Autodesk Inventor part; units mm, degrees
ref_plane "Work Plane1" through (-39.4462, 0, -3.175) normal (0, 0, -1) x (0, 1, 0)
ref_plane "YZ Plane" through (0, 0, 0) normal (1, 0, 0) x (0, 1, 0)
ref_plane "XZ Plane" through (0, 0, 0) normal (0, 1, 0) x (-1, 0, 0)
sketch "Sketch1" plane through (0, 0, 0) normal (0, 0, 1) x (1, 0, 0)
  line L0 (-43.688, 0) -> (-43.688, 415.3)
  line L1 (0, 0) -> (0, 415.3)
  circle A0 centre (-7.6009, 150.0066) radius 1.1
  circle A1 centre (-13.6588, 173.1577) radius 6.4135
  circle A2 centre (-13.6588, 134.9467) radius 6.4135
  circle A3 centre (-7.6009, 188.2176) radius 1.1
  circle A4 centre (-7.6009, 92.9676) radius 1.1
  circle A5 centre (-13.6588, 245.4367) radius 6.4135
  circle A6 centre (-13.6588, 77.9077) radius 6.4135
  circle A7 centre (-7.6009, 260.4966) radius 1.1
  circle A8 centre (-7.6009, 54.7566) radius 1.1
  circle A9 centre (-13.6588, 283.6477) radius 6.4135
  circle A10 centre (-13.6588, 39.6967) radius 6.4135
  circle A11 centre (-7.6009, 298.7076) radius 1.1
  line L2 (-7.3698, 0) -> (-7.3698, 12.7)
  line L3 (-7.3698, 0) -> (-36.3182, 0)
  line L4 (-36.3182, 0) -> (-36.3182, 12.7)
  line L5 (-36.3182, 12.7) -> (-39.4462, 12.7)
  line L6 (-39.4462, 12.7) -> (-39.4462, 402.6)
  line L7 (-39.4462, 402.6) -> (-36.3182, 402.6)
  line L8 (-36.3182, 402.6) -> (-36.3182, 415.3)
  line L9 (-36.3182, 415.3) -> (-7.3698, 415.3)
  line L10 (-7.3698, 402.6) -> (-7.3698, 415.3)
  line L11 (-7.3698, 402.6) -> (-4.2418, 402.6)
  line L12 (-4.2418, 402.6) -> (-4.2418, 12.7)
  line L13 (-4.2418, 12.7) -> (-7.3698, 12.7)
  circle A12 centre (-13.6588, 340.6867) radius 6.4135
  circle A13 centre (-7.6009, 355.7466) radius 1.1
  circle A14 centre (-13.6588, 378.8977) radius 6.4135
  circle A15 centre (-34.9052, 110.3753) radius 3.2004
  circle A16 centre (-34.9052, 316.1153) radius 3.2004
  circle A17 centre (-7.6009, 393.9576) radius 1.1
  circle A18 centre (-11.9075, 15.1253) radius 3.302
  circle A19 centre (-23.6029, 54.7566) radius 1.1
  circle A20 centre (-23.6029, 92.9676) radius 1.1
  circle A21 centre (-23.6029, 188.2176) radius 1.1
  circle A22 centre (-23.6029, 260.4966) radius 1.1
  circle A23 centre (-34.9052, 322.1732) radius 1.1
  circle A24 centre (-23.6029, 355.7466) radius 1.1
  circle A25 centre (-23.6029, 393.9576) radius 1.1
  circle A26 centre (-23.6029, 298.7076) radius 1.1
  circle A27 centre (-23.6029, 150.0066) radius 1.1
  circle A28 centre (-34.9052, 116.4332) radius 1.1
  circle A29 centre (-11.9075, 316.1153) radius 3.302
  circle A30 centre (-13.6588, 328.1211) radius 3.302
  circle A31 centre (-13.6588, 366.3321) radius 3.302
  circle A32 centre (-13.6588, 271.0821) radius 3.302
  circle A33 centre (-13.6588, 232.8711) radius 3.302
  circle A34 centre (-29.6608, 160.5921) radius 3.302
  circle A35 centre (-29.6608, 122.3811) radius 3.302
  circle A36 centre (-11.9075, 110.3753) radius 3.302
  circle A37 centre (-13.6588, 65.3421) radius 3.302
  circle A38 centre (-13.6588, 27.1311) radius 3.302
  circle A39 centre (-29.6608, 27.1311) radius 3.302
  circle A40 centre (-29.6608, 65.3421) radius 3.302
  circle A41 centre (-13.6588, 122.3811) radius 3.302
  circle A42 centre (-13.6588, 160.5921) radius 3.302
  circle A43 centre (-11.9075, 220.8653) radius 3.302
  circle A44 centre (-29.6608, 232.8711) radius 3.302
  circle A45 centre (-29.6608, 271.0821) radius 3.302
  circle A46 centre (-29.6608, 366.3321) radius 3.302
  circle A47 centre (-29.6608, 328.1211) radius 3.302
  circle A48 centre (-29.6583, 340.6867) radius 6.4135
  circle A49 centre (-29.6583, 378.8977) radius 6.4135
  circle A50 centre (-29.6583, 245.4367) radius 6.4135
  circle A51 centre (-29.6583, 173.1577) radius 6.4135
  circle A52 centre (-29.6583, 134.9467) radius 6.4135
  circle A53 centre (-29.6583, 39.6967) radius 6.4135
  circle A54 centre (-29.6583, 77.9077) radius 6.4135
  circle A55 centre (-29.6583, 283.6477) radius 6.4135
  circle A56 centre (-22.9108, 110.3753) radius 4.5
  circle A57 centre (-22.9108, 220.8653) radius 4.5
  circle A58 centre (-22.9108, 316.1153) radius 4.5
  circle A59 centre (-13.6588, 355.7466) radius 3.2004
  circle A60 centre (-29.6608, 393.9576) radius 3.2004
  circle A61 centre (-29.6608, 298.7076) radius 3.2004
  circle A62 centre (-13.6588, 260.4966) radius 3.2004
  circle A63 centre (-13.6588, 188.2176) radius 3.2004
  circle A64 centre (-13.6588, 150.0066) radius 3.2004
  circle A65 centre (-13.6588, 92.9676) radius 3.2004
  circle A66 centre (-29.6608, 54.7566) radius 3.2004
  circle A67 centre (-13.6588, 54.7566) radius 3.2004
  circle A68 centre (-29.6608, 92.9676) radius 3.2004
  circle A69 centre (-29.6608, 150.0066) radius 3.2004
  circle A70 centre (-29.6608, 188.2176) radius 3.2004
  circle A71 centre (-29.6608, 260.4966) radius 3.2004
  circle A72 centre (-13.6588, 298.7076) radius 3.2004
  circle A73 centre (-13.6588, 393.9576) radius 3.2004
  circle A74 centre (-29.6608, 355.7466) radius 3.2004
  circle A75 centre (-21.844, 200.6606) radius 6.25
  circle A76 centre (-21.844, 406.4006) radius 6.25
  circle A77 centre (-22.9108, 15.1253) radius 4.5
  line L14 (-36.3182, 0) -> (-43.688, 0)
  line L15 (0, 0) -> (-7.3698, 0)
  line L16 (0, 5.79) -> (-43.688, 5.79)
  line L17 (0, 212.165) -> (-43.688, 212.165)
  dimension "d0" = 206.375
ref_plane "Work Plane1" through (-39.4462, 0, -3.175) normal (0, 0, -1) x (0, 1, 0)
extrude "Extrusion1" add sketch "Sketch1" against normal up to surface (3.175 mm away) contours L0 L17 L6 L5 L4 L16 | L4 L5 L6 L17 L12 L13 L2 L16 | L2 L13 L12 L17 L1 L16
properties part number "HalfInterlockBox"
Build history of the part. All positions in model axes, mm. Round coordinates to 2 decimals unless told otherwise and drop trailing zeros. Loops run counter-clockwise (first coordinate to the right, second up) from the corner with the lowest first, then second, coordinate; pieces in that order, holes last. Notation, with made-up numbers: (9.5, -40) -> (14.5, -40) arc R6 cw to (14.5, -31) -> close; hole circle Ø1 at (75, -20). An arc over 180 degrees is marked (long way). One line per item, written item: value. Start each with the question number.
Q1. Two-plate mould, pull along X, no slides. Class faces 1 (the face through (-18.62, 16.48, -1.57)), 2 (the face through (-26.699, 72.218, -1.565)), 3 (the face through (-43.688, 108, -2)), 4 (the face through (-22, 212.165, -2)): released by +X, released by -X, zero draft, split by the parting line, or undercut.
Q2. Drop flat-ended pins along their axis: pin 1 Ø12 at (x, y) = (-33.5, 121.5) entering from +Z; pin 2 Ø1.8 at (x, y) = (-23.6, 54.76) entering from -Z. Give the stop position or say it passes through.
Q3. Probe line 1 along X through (y, z) = (110, -1.5); line 2 along X through (y, z) = (161, -1.15); line 3 along X through (y, z) = (188.5, -0.25). List the from-to ranges inside material, lowest first.
Q4. Cut at B-B on z = -1.2. Count the separate pieces of the cut face and the enclosed holes in it, plus the area to 3 significant figures.
Q5. Cut at A-A on y = 198.5. List the corners of the cut face in (x, z) (3 decimals).
Computed:
1. face 1: undercut
1. face 2: undercut
1. face 3: released by -X
1. face 4: zero draft
2. pin 1: z = 0
2. pin 2: through
3. line 1: -43.69 to -38.08, -31.73 to -27.4, -18.43 to -15.19, -8.63 to 0
3. line 2: -43.69 to -32.94, -26.38 to -16.94, -10.38 to 0
3. line 3: -43.69 to -32.85, -26.47 to -24.67, -22.54 to -16.85, -10.47 to -8.66, -6.54 to 0
4. separate pieces: 1
4. enclosed holes: 39
4. area: 7,070 mm²
5. outline: (-43.688, -3.175) -> (-27.709, -3.175) -> (-27.709, 0) -> (-43.688, 0) -> close; (-15.979, -3.175) -> (0, -3.175) -> (0, 0) -> (-15.979, 0) -> close
